Model file for the job. Use its own axes, mm. Face numbers are marked on the shaded views. A direction names the side the tool comes from. Coordinates: 2 decimals unless noted, no trailing zeros. Order: outer loops, then holes, each group sorted by start corner. A loop starts at its lowest first (then second) coordinate and runs counter-clockwise, first axis right, second up. Notation, with made-up numbers: (9, 77) -> (16, 77) arc R30 cw to (16, 115) -> close; hole circle Ø11 at (23, 6). An arc over 180 degrees is marked (long way). Return JSON: item names as keys, results as strings. Group by question number.
1) Cut at C-C (y = 3.5). Write the cut outline in (x, z).
2) Which spindle directions (+Z, -Z, +X, -X, +Y, -Y) get a long thin tool onto all of the face, cutting with end or side? Do the marked faces 1, 2, 3, 4 and 5. Say none if no direction does.
3) Cut at A-A (z = 3.25). Write the cut outline in (x, y).
4) Flat gauge pins, fed straight in: pin 1 (0.6 mm diameter, centred on x = 10.5, y = 0, fed in from -Z); pin 2 (0.8 mm diameter, centred on x = 10.5, z = 3.5, fed in from -Y); pin 3 (1.1 mm diameter, centred on x = 10.5, z = 3.5, fed in from +Y). Where does each tip first touch, or does it go through?
5) Cut at B-B (x = -1.5). Write the cut outline in (y, z), and give its area (3 significant figures).
6) Cut at D-D (y = -6). Write the cut outline in (x, z).
7) Probe line 1 (Y direction, x = 0, z = -0.8); line 2 (Y direction, x = 0, z = 9.25); line 3 (X direction, y = 10.5, z = 10). List the from-to ranges inside material, lowest first.
8) Pull direction X, two halves, no side cores. Call the marked faces 6, 7 and 8: +X half, -X half, draft (parallel to the pull), parting line (faces both ways), or undercut.
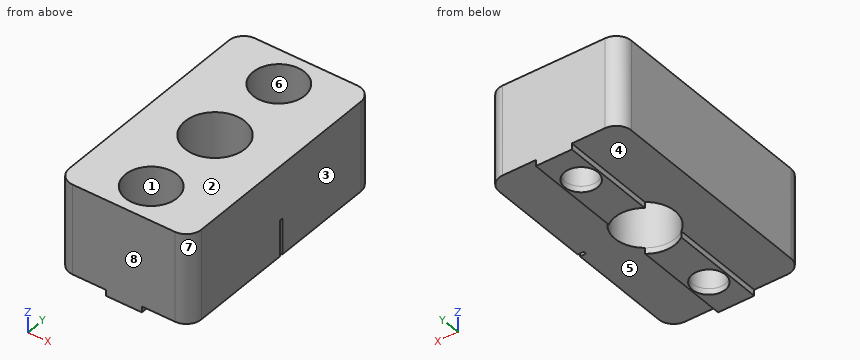
from build123d import *

# Parameters (mm, degrees)
F1_W      = 22
F1_H      = 40
F1_R      = 2.75
F1_R_2    = 5
F2_DEPTH  = 15
F3_R      = 4.3
F4_DEPTH  = 11
F5_R      = 2.5
F6_R      = 2.75
F7_DEPTH  = 1
F8_R      = 2.75
F9_DEPTH  = 0.3
F10_W     = 0.25
F10_H     = 6
F11_DEPTH = 1


with BuildPart() as f2:
    # F1 (on Top) → F2 (new body)
    with BuildSketch(Plane.XY):
        Rectangle(F1_W, F1_H)
        with Locations((0, -14)):
            Circle(F1_R, mode=Mode.SUBTRACT)
        Circle(F1_R_2, mode=Mode.SUBTRACT)
        with Locations((0, 14)):
            Circle(F1_R, mode=Mode.SUBTRACT)
    extrude(amount=F2_DEPTH)

    # F3 (on face) → F4 (cut)
    with BuildSketch(Plane.XY.offset(15)):
        with Locations((0, 14)):
            Circle(F3_R)
        with Locations((0, -14)):
            Circle(F3_R)
    extrude(amount=-F4_DEPTH, mode=Mode.SUBTRACT)

    # F5
    f5_edges = [f2.edges().sort_by_distance(p)[0] for p in [
        (11, -20, 7.5),
        (-11, -20, 7.5),
        (11, 20, 7.5),
        (-11, 20, 7.5),
    ]]
    fillet(f5_edges, radius=F5_R)

    # F6 (on face) → F7 (join)
    with BuildSketch(Plane.XY):
        with BuildLine():
            Line((-3, -20), (0, -20))
            Line((0, -20), (3, -20))
            Line((3, -20), (3, -4))
            ThreePointArc((3, -4), (0, -5), (-3, -4))
            Line((-3, -4), (-3, -20))
        make_face()
        with Locations((0, -14)):
            Circle(F6_R, mode=Mode.SUBTRACT)
        with BuildLine():
            Line((3, 20), (0, 20))
            Line((0, 20), (-3, 20))
            Line((-3, 20), (-3, 4))
            ThreePointArc((-3, 4), (0, 5), (3, 4))
            Line((3, 4), (3, 20))
        make_face()
        with Locations((0, 14)):
            Circle(F6_R, mode=Mode.SUBTRACT)
    extrude(amount=-F7_DEPTH)

    # F8 (on face) → F9 (join)
    with BuildSketch(Plane.XY.offset(4)):
        with Locations((0, 14)):
            Circle(F8_R)
        with Locations((0, -14)):
            Circle(F8_R)
    extrude(amount=-F9_DEPTH)

    # F10 (on face) → F11 (cut)
    with BuildSketch(Plane.YZ.offset(11)):
        with Locations((0.125, 3)):
            Rectangle(F10_W, F10_H)
        with Locations((-0.125, 3)):
            Rectangle(F10_W, F10_H)
    extrude(amount=-F11_DEPTH, mode=Mode.SUBTRACT)


solid = f2.part
Answers below:
{
 "1": {"outline": "(-11, 0) -> (-3.57, 0) -> (-3.57, 15) -> (-11, 15) -> close; (3.57, 0) -> (11, 0) -> (11, 15) -> (3.57, 15) -> close"},
 "2": {"face 1": "+Z", "face 2": "+Z, +X, -X, +Y, -Y", "face 3": "+Z, -Z, +X, +Y, -Y", "face 4": "-Z, -X, +Y, -Y", "face 5": "-Z, +X, +Y, -Y"},
 "3": {"outline": "(-11, -17.5) arc R2.5 ccw to (-8.5, -20) -> (8.5, -20) arc R2.5 ccw to (11, -17.5) -> (11, -0.25) -> (10, -0.25) -> (10, 0.25) -> (11, 0.25) -> (11, 17.5) arc R2.5 ccw to (8.5, 20) -> (-8.5, 20) arc R2.5 ccw to (-11, 17.5) -> close; hole circle Ø10 at (0, 0); hole circle Ø5.5 at (0, -14); hole circle Ø5.5 at (0, 14)"},
 "4": {"pin 1": "stops at z = 0", "pin 2": "stops at y = -19.42", "pin 3": "stops at y = 19.54"},
 "5": {"outline": "(-20, -1) -> (-16.3, -1) -> (-16.3, 3.7) -> (-11.7, 3.7) -> (-11.7, -1) -> (-4.77, -1) -> (-4.77, 15) -> (-9.97, 15) -> (-9.97, 4) -> (-18.03, 4) -> (-18.03, 15) -> (-20, 15) -> close; (4.77, -1) -> (11.7, -1) -> (11.7, 3.7) -> (16.3, 3.7) -> (16.3, -1) -> (20, -1) -> (20, 15) -> (18.03, 15) -> (18.03, 4) -> (9.97, 4) -> (9.97, 15) -> (4.77, 15) -> close", "area": "267 mm^2"},
 "6": {"outline": "(-11, 0) -> (-3, 0) -> (-3, -1) -> (3, -1) -> (3, 0) -> (11, 0) -> (11, 15) -> (-11, 15) -> close"},
 "7": {"line 1": "y = -20 to -16.75, -11.25 to -5, 5 to 11.25, 16.75 to 20", "line 2": "y = -20 to -18.3, -9.7 to -5, 5 to 9.7, 18.3 to 20", "line 3": "x = -11 to -2.5, 2.5 to 11"},
 "8": {"face 6": "undercut", "face 7": "+X half", "face 8": "draft"}
}
